Source: CAD feature listing. Evaluate the final solid. Frame: model axes, mm. A direction names the side the tool comes from. Round coordinates to 2 decimals unless told otherwise and drop trailing zeros. Write each loop counter-clockwise with the first axis right and the second up, starting at its lowest first coordinate (ties: lowest second). Pieces come first, ordered by that corner, then holes.
Solid Edge part; units mm, degrees
sketch "Sketch1" plane through (0, 0, 0) normal (0, 0, 1) x (1, 0, 0)
  line L0 (26, -14.5) -> (26, 14.5)
  line L1 (26, 14.5) -> (-26, 14.5)
  line L2 (-26, 14.5) -> (-26, -14.5)
  line L3 (-26, -14.5) -> (26, -14.5)
extrude "Protrusion1" add sketch "Sketch1" along normal blind 1.5
sketch "Sketch2" plane through (0, 0, 1.5) normal (0, 0, 1) x (1, 0, 0)
  line L0 (-14, 12.1) -> (21, 12.1)
  line L1 (21, 12.1) -> (21, 14.5)
  line L2 (21, 14.5) -> (-14, 14.5)
  line L3 (-14, 14.5) -> (-14, 12.1)
  line L4 (21, -14.5) -> (21, -12.1)
  line L5 (21, -12.1) -> (-14, -12.1)
  line L6 (-14, -12.1) -> (-14, -14.5)
  line L7 (-14, -14.5) -> (21, -14.5)
extrude "ExtrudedProtrusion_2" add sketch "Sketch2" along normal blind 8
sketch "Sketch3" plane through (0, 0, 0) normal (0, 0, -1) x (-1, 0, 0)
  line L0 (-19, -8.5) -> (-1, -8.5)
  line L1 (-1, -8.5) -> (-1, 7.5)
  line L2 (-1, 7.5) -> (-19, 7.5)
  line L3 (-19, 7.5) -> (-19, -8.5)
extrude "ExtrudedProtrusion_3" add sketch "Sketch3" along normal blind 3.4
sketch "Sketch4" plane through (0, 0, 0) normal (0, 0, -1) x (-1, 0, 0)
  line L0 (26, 4.5) -> (20.6, 4.5)
  line L1 (20.6, 4.5) -> (20.6, -2.9)
  line L2 (20.6, -2.9) -> (26, -2.9)
  line L3 (26, -2.9) -> (26, 4.5)
extrude "ExtrudedProtrusion_4" add sketch "Sketch4" along normal blind 2.5
properties material "ABS Plastic, high impact"
1) Contact query for flat-ended pins moving along their axis: P1, Ø0.8, axis at y = -0.5, z = -1.5, coming from the +X side; P2, Ø4, axis at x = 16, y = 8.5, coming from the +Z side; P3, Ø1.9, axis at y = -13, z = 6, coming from the -X side. Output: stop coordinate, or through.
Taken from the geometry:
P1: stops at x = 19
P2: stops at z = 1.5
P3: stops at x = -14
2) Material intervals for line 1 (Y direction, x = -2, z = 4); line 2 (X direction, y = -12.75, z = 1.75); line 3 (X direction, y = -0.5, z = -2), sorted ascending.
Taken from the geometry:
line 1: y = -14.5 to -12.1, 12.1 to 14.5
line 2: x = -14 to 21
line 3: x = -26 to -20.6, 1 to 19
3) Pull-direction query (Y, two-part tool) for faces 5 (the face through (3, 12.1, 5)), 6 (the face through (-23, -2.9, -1)), 7 (the face through (3, -13, 9.5)); classes: released by +Y, released by -Y, zero draft, split by the parting line, or undercut.
Taken from the geometry:
face 5: undercut
face 6: released by -Y
face 7: zero draft
4) Section query C-C on x = 15. Return the cut outline in (y, z).
Taken from the geometry:
outline: (-14.5, 0) - (-8.5, 0) - (-8.5, -3.4) - (7.5, -3.4) - (7.5, 0) - (14.5, 0) - (14.5, 9.5) - (12.1, 9.5) - (12.1, 1.5) - (-12.1, 1.5) - (-12.1, 9.5) - (-14.5, 9.5) - close
5) Section query B-B on y = -6.5. Return the cut outline in (x, z).
Taken from the geometry:
outline: (-26, 0) - (1, 0) - (1, -3.4) - (19, -3.4) - (19, 0) - (26, 0) - (26, 1.5) - (-26, 1.5) - close
6) Reachability of faces 1 (the face through (4, -12.1, 5)), 2 (the face through (10, 7.5, -2)), 3 (the face through (10, -8.5, -2)), 4 (the face through (-20.6, 1, -1)) from +Z, -Z, +X, -X, +Y, -Y: full face, straight path, thin tool, end or side. Return the list, or none.
Taken from the geometry:
face 1: +Z, +X, -X
face 2: -Z, +X, -X, +Y
face 3: -Z, +X, -X, -Y
face 4: -Z, +Y, -Y
7) Section query A-A on z = 4.25. Return the cut outline in (x, y), then the cut area to 3 significant figures.
Taken from the geometry:
outline: (-14, -14.5) - (21, -14.5) - (21, -12.1) - (-14, -12.1) - close; (-14, 12.1) - (21, 12.1) - (21, 14.5) - (-14, 14.5) - close
area: 168 mm2
8) Section query D-D on x = -3. Return the cut outline in (y, z), then the cut area to 3 significant figures.
Taken from the geometry:
outline: (-14.5, 0) - (14.5, 0) - (14.5, 9.5) - (12.1, 9.5) - (12.1, 1.5) - (-12.1, 1.5) - (-12.1, 9.5) - (-14.5, 9.5) - close
area: 81.9 mm2
